Check sheet for the drawn part. Datum: minimum x, y, z corner. Units: mm. Coordinates: 2 decimals unless noted, no trailing zeros. Write each loop counter-clockwise with the first axis right and the second up, starting at its lowest first coordinate (ties: lowest second). Pieces come first, ordered by that corner, then holes. Notation, with made-up numbers: (54, -28.5) - (77, -28.5) arc R25 ccw to (77, 4.5) - close; hole circle Ø2 at (-28, 51). An arc over 180 degrees is marked (long way). Answer as CSV lines item,"result". Start each with the question number.
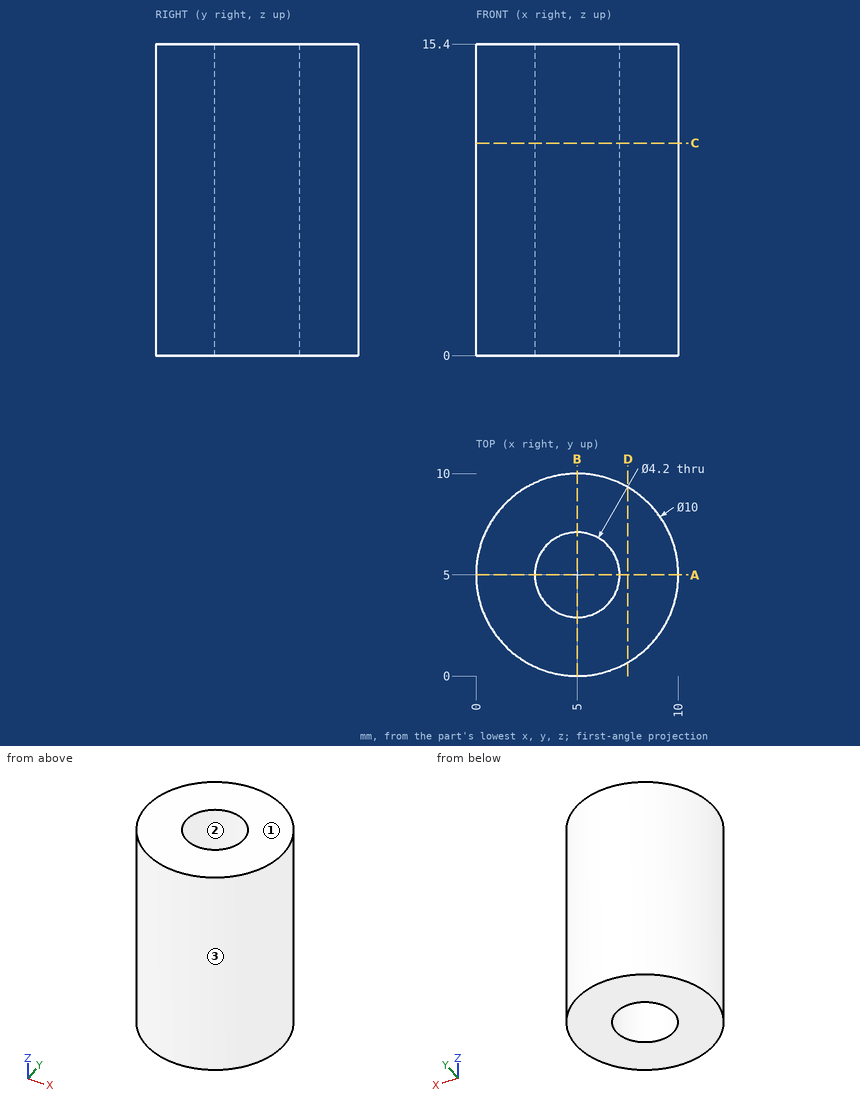
(1) Material ranges on probe 1 along Y at (x, z) = (5, 6.25); probe 2 along Y at (x, z) = (5.75, 7.25); probe 3 along X at (y, z) = (6.25, 8), recorded low to high. Write a range as from..to.
(2) Cross-section at A-A on y = 5. Record the boundary of the cut face in (x, z), plus the area to 3 significant figures.
(3) Cross-section at C-C on z = 10.5. Record the boundary of the cut face in (x, y), plus the area to 3 significant figures.
(4) Cross-section at D-D on x = 7.5. Record the boundary of the cut face in (y, z), plus the area to 3 significant figures.
(5) Release check for a two-part mould opening along X. For the marked faces 1, 2 and 3 record: pulls with the +X half, pulls with the -X half, needs draft (parallel to the pull), parting line crosses it, or undercut.
(6) Go/stop test with flat-tipped pins: P1, Ø2, axis at x = 6.5, z = 9.5, coming from the -Y side; P2, Ø1.5, axis at x = 1, z = 10.5, coming from the +Y side; P3, Ø4, axis at x = 5, y = 5, coming from the +Z side. Record where each tip stops, or that it passes through.
Checked values:
1,probe 1,"0..2.9, 7.1..10"
1,probe 2,"0.06..3.04, 6.96..9.94"
1,probe 3,"0.16..3.31, 6.69..9.84"
2,outline,"(0, 0) - (2.9, 0) - (2.9, 15.4) - (0, 15.4) - close; (7.1, 0) - (10, 0) - (10, 15.4) - (7.1, 15.4) - close"
2,area,"89.3 mm^2"
3,outline,"circle Ø10 at (5, 5); hole circle Ø4.2 at (5, 5)"
3,area,"64.7 mm^2"
4,outline,"(0.67, 0) - (9.33, 0) - (9.33, 15.4) - (0.67, 15.4) - close"
4,area,"133 mm^2"
5,face 1,"needs draft"
5,face 2,"undercut"
5,face 3,"parting line crosses it"
6,P1,"y = 0.03"
6,P2,"y = 8.8"
6,P3,"through"
